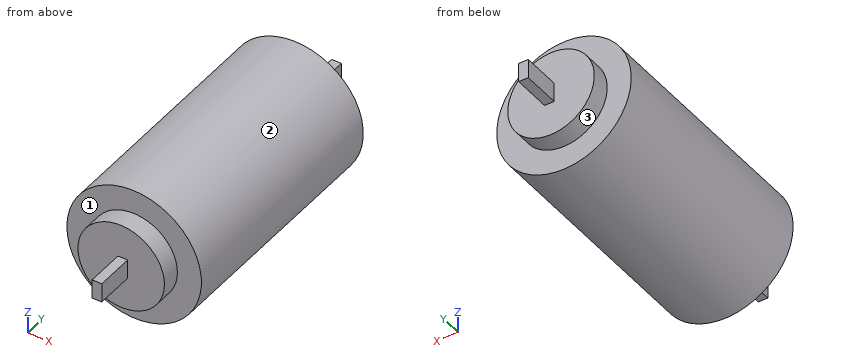
Autodesk Inventor part; units mm, degrees
ref_plane "YZ Plane" through (0, 0, 0) normal (1, 0, 0) x (0, 1, 0)
ref_plane "XZ Plane" through (0, 0, 0) normal (0, 1, 0) x (-1, 0, 0)
ref_plane "XY Plane" through (0, 0, 0) normal (0, 0, 1) x (1, 0, 0)
sketch "Sketch1" plane through (0, 0, 0) normal (0, 1, 0) x (-1, 0, 0)
  circle A0 centre (0, 0) radius 7
  dimension "d0" = 14
extrude "Extrusion1" add sketch "Sketch1" along normal blind 25
sketch "Sketch2" plane through (0, 25, 0) normal (0, 1, 0) x (1, 0, 0)
  circle A0 centre (0, 0) radius 4.5
  dimension "d3" = 9
sketch "Sketch3" plane through (0, 0, 0) normal (0, -1, 0) x (1, 0, 0)
  circle A0 centre (0, 0) radius 4.5
  dimension "d4" = 9
extrude "Extrusion2" add sketch "Sketch3" along normal mid plane 4
extrude "Extrusion3" add sketch "Sketch2" along normal blind 2
sketch "Sketch4" plane through (0, -2, 0) normal (0, -1, 0) x (1, 0, 0)
  line L0 (-0.3275, -1.0042) -> (0.6725, -1.0042)
  line L1 (0.6725, -1.0042) -> (0.6725, 0.9958)
  line L2 (0.6725, 0.9958) -> (-0.3275, 0.9958)
  line L3 (-0.3275, 0.9958) -> (-0.3275, -1.0042)
  point P0 (0, 0)
  dimension "d9" = 1
  dimension "d10" = 2
extrude "Extrusion4" add sketch "Sketch4" along normal blind 4
sketch "Sketch5" plane through (0, 27, 0) normal (0, 1, 0) x (1, 0, 0)
  line L0 (0.6725, -0.9958) -> (-0.3275, -0.9958)
  line L1 (0.6725, 1.0042) -> (0.6725, -0.9958)
  line L2 (-0.3275, -0.9958) -> (0.6725, -0.9958)
  line L3 (0.6725, -0.9958) -> (0.6725, 1.0042)
  line L4 (0.6725, 1.0042) -> (-0.3275, 1.0042)
  line L5 (-0.3275, 1.0042) -> (-0.3275, -0.9958)
  point P0 (0, 0)
extrude "Extrusion5" add sketch "Sketch5" along normal blind 4
properties part number "tilt"
Verification items for the finished model (mm, model axes). Face numbers are marked on the shaded views. A direction names the side the tool comes from. Round coordinates to 2 decimals unless told otherwise and drop trailing zeros. Write each loop counter-clockwise with the first axis right and the second up, starting at its lowest first coordinate (ties: lowest second). Pieces come first, ordered by that corner, then holes.
1. Gauge pin test, flat ends, axial feed: P1, Ø0.8, axis at x = 0, y = -5, coming from the +Z side; P2, Ø1, axis at x = 2.5, z = 2, coming from the -Y side; P3, Ø1.6, axis at y = -4, z = 0, coming from the +X side. Record the tip position at first contact, or that the pin passes through.
2. Section check A-A on z = 0. Enter the section's corners in (x, y), plus the area to 3 significant figures.
3. Section check C-C on y = 11. Enter the section's corners in (x, z).
4. Scan lines: L1, parallel to Y at x = -1.5, z = -1.25; L2, parallel to Z at x = 0.5, y = 28; L3, parallel to Y at x = -5.5, z = 0.75. Record each from-to range of solid material in increasing order.
5. Section check D-D on x = -3.75. Enter the section's corners in (y, z), plus the area to 3 significant figures.
6. Access from +Z, -Z, +X, -X, +Y, -Y to the whole of each face (thin tool, end or side, straight path). Record for the marked faces 1, 2 and 3.
7. Section check B-B on x = 3. Enter the section's corners in (y, z), plus the area to 3 significant figures.
Answer:
1. P1: stops at z = 1
1. P2: stops at y = -2
1. P3: stops at x = 0.67
2. outline: (-7, 0) - (-4.5, 0) - (-4.5, -2) - (-0.33, -2) - (-0.33, -6) - (0.67, -6) - (0.67, -2) - (4.5, -2) - (4.5, 0) - (7, 0) - (7, 25) - (4.5, 25) - (4.5, 27) - (0.67, 27) - (0.67, 31) - (-0.33, 31) - (-0.33, 27) - (-4.5, 27) - (-4.5, 25) - (-7, 25) - close
2. area: 394 mm2
3. outline: circle Ø14 at (0, 0)
4. L1: y = -2 to 27
4. L2: z = -1 to 1
4. L3: y = 0 to 25
5. outline: (-2, -2.49) - (0, -2.49) - (0, -5.91) - (25, -5.91) - (25, -2.49) - (27, -2.49) - (27, 2.49) - (25, 2.49) - (25, 5.91) - (0, 5.91) - (0, 2.49) - (-2, 2.49) - close
5. area: 315 mm2
6. face 1: -Y
6. face 2: +Y, -Y
6. face 3: +Y
7. outline: (-2, -3.35) - (0, -3.35) - (0, -6.32) - (25, -6.32) - (25, -3.35) - (27, -3.35) - (27, 3.35) - (25, 3.35) - (25, 6.32) - (0, 6.32) - (0, 3.35) - (-2, 3.35) - close
7. area: 343 mm2
